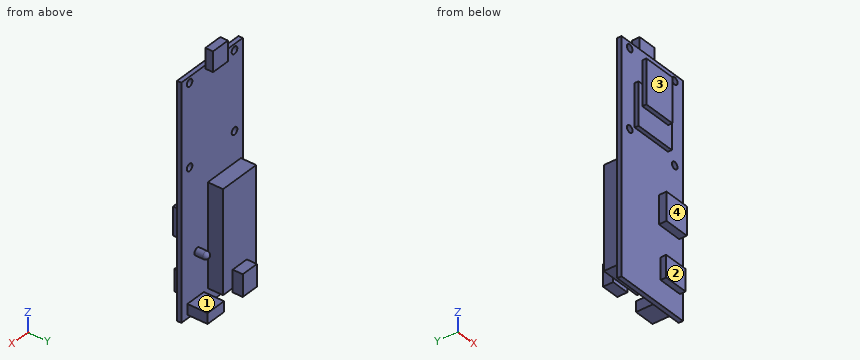
Autodesk Inventor part; units mm, degrees
ref_plane "YZ Plane" through (0, 0, 0) normal (1, 0, 0) x (0, 1, 0)
ref_plane "XZ Plane" through (0, 0, 0) normal (0, 1, 0) x (-1, 0, 0)
ref_plane "XY Plane" through (0, 0, 0) normal (0, 0, 1) x (1, 0, 0)
sketch "Sketch1" plane through (0, 0, 0) normal (0, 1, 0) x (-1, 0, 0)
  line L0 (16.375, 48.6) -> (-16.375, 48.6)
  line L1 (-16.375, 48.6) -> (-16.375, -48.6)
  line L2 (-16.375, -48.6) -> (16.375, -48.6)
  line L3 (16.375, -48.6) -> (16.375, 48.6)
  line L4 (16.375, 48.6) -> (-16.375, -48.6) construction
  line L5 (-16.375, 48.6) -> (16.375, -48.6) construction
  point P0 (0, 0)
  dimension "d0" = 32.75
  dimension "d1" = 97.2
extrude "Extrusion1" add sketch "Sketch1" along normal blind 1.8
sketch "Sketch4" plane through (0, 0, 0) normal (0, -1, 0) x (1, 0, 0)
  line L0 (8.375, 33.45) -> (-9.375, 33.45)
  line L1 (-9.375, 33.45) -> (-9.375, 15.45)
  line L2 (-9.375, 15.45) -> (8.375, 15.45)
  line L3 (8.375, 15.45) -> (8.375, 33.45)
  line L4 (16.375, 48.6) -> (16.375, -48.6)
  line L5 (-16.375, 48.6) -> (16.375, 48.6)
  point P0 (0, 0)
  dimension "d12" = 18
  dimension "d13" = 17.75
  dimension "d14" = 8
  dimension "d15" = 15.15
extrude "Extrusion4" add sketch "Sketch4" along normal blind 3.43 from surface at -1.8
sketch "Sketch5" plane through (-9.375, -1.63, 33.45) normal (0, -1, 0) x (1, 0, 0)
  line L0 (2, -9) -> (15.8, -9)
  line L1 (15.8, -9) -> (15.8, 9.6)
  line L2 (15.8, 9.6) -> (2, 9.6)
  line L3 (2, 9.6) -> (2, -9)
  line L4 (0, 0) -> (0, -18)
  line L5 (0, -18) -> (17.75, -18)
  point P0 (9.375, -33.45)
  dimension "d18" = 18.6
  dimension "d19" = 13.8
  dimension "d20" = 2
  dimension "d21" = 9
extrude "Extrusion5" add sketch "Sketch5" along normal blind 1.75 from surface at 0
sketch "Sketch6" plane through (0, 0, 0) normal (0, -1, 0) x (1, 0, 0)
  line L0 (14.375, -4.75) -> (3.525, -4.75)
  line L1 (3.525, -4.75) -> (3.525, -16.6)
  line L2 (3.525, -16.6) -> (14.375, -16.6)
  line L3 (14.375, -16.6) -> (14.375, -4.75)
  line L4 (16.375, 48.6) -> (16.375, -48.6)
  line L5 (16.375, -48.6) -> (-16.375, -48.6)
  point P0 (0, 0)
  dimension "d24" = 11.85
  dimension "d25" = 10.85
  dimension "d26" = 2
  dimension "d27" = 32
extrude "Extrusion6" add sketch "Sketch6" along normal blind 5.04 from surface at -1.8
sketch "Sketch7" plane through (0, 0, 0) normal (0, -1, 0) x (1, 0, 0)
  line L0 (14.775, -29.45) -> (4.445, -29.45)
  line L1 (4.445, -29.45) -> (4.445, -38.6)
  line L2 (4.445, -38.6) -> (14.775, -38.6)
  line L3 (14.775, -38.6) -> (14.775, -29.45)
  line L4 (16.375, 48.6) -> (16.375, -48.6)
  line L5 (16.375, -48.6) -> (-16.375, -48.6)
  point P0 (0, 0)
  dimension "d30" = 9.15
  dimension "d31" = 10.33
  dimension "d32" = 1.6
  dimension "d33" = 10
extrude "Extrusion7" add sketch "Sketch7" along normal blind 4.18 from surface at -1.8
sketch "Sketch8" plane through (0, 1.8, 0) normal (0, 1, 0) x (1, 0, 0)
  line L0 (-4.375, -47.18) -> (3.555, -47.18)
  line L1 (3.555, -47.18) -> (3.555, -55.6)
  line L2 (3.555, -55.6) -> (-4.375, -55.6)
  line L3 (-4.375, -55.6) -> (-4.375, -47.18)
  line L4 (-16.375, 48.6) -> (-16.375, -48.6)
  line L5 (-16.375, -48.6) -> (16.375, -48.6)
  point P0 (0, 0)
  dimension "d36" = 8.42
  dimension "d37" = 7.93
  dimension "d38" = 12
  dimension "d39" = 7
extrude "Extrusion8" add sketch "Sketch8" along normal blind 3.23
sketch "Sketch9" plane through (0, 1.8, 0) normal (0, 1, 0) x (1, 0, 0)
  circle A0 centre (-11.975, -46.1) radius 1.5
  circle A1 centre (11.975, -46.1) radius 1.5
  circle A2 centre (11.975, -11.9) radius 1.5
  circle A3 centre (-11.975, -13.4) radius 1.5
  line L0 (-13.475, -13.4) -> (-16.375, -13.4)
  line L1 (-16.375, 48.6) -> (-16.375, -48.6)
  line L2 (-13.475, -13.4) -> (-11.975, -13.4) construction
  line L3 (-11.975, -46.1) -> (-13.475, -46.1) construction
  line L4 (-13.475, -46.1) -> (-16.375, -46.1)
  line L5 (-11.975, -46.1) -> (-11.975, -47.6) construction
  line L6 (-16.375, -48.6) -> (16.375, -48.6)
  line L7 (-11.975, -47.6) -> (-11.975, -48.6)
  line L8 (11.975, -46.1) -> (13.475, -46.1) construction
  line L9 (13.475, -46.1) -> (16.375, -46.1)
  line L10 (11.975, -46.1) -> (11.975, -47.6) construction
  line L11 (11.975, -47.6) -> (11.975, -48.6)
  line L12 (16.375, -48.6) -> (16.375, 48.6)
  line L13 (11.975, -46.1) -> (11.975, -44.6) construction
  line L14 (11.975, -44.6) -> (11.975, -13.4)
  line L15 (11.975, -13.4) -> (11.975, -11.9) construction
  line L16 (-11.975, -46.1) -> (-11.975, -14.9)
  line L17 (-11.975, -13.4) -> (-11.975, -14.9) construction
  point P0 (0, 0)
  dimension "d42" = 3
  dimension "d43" = 2.9
  dimension "d44" = 2.9
  dimension "d45" = 1
  dimension "d46" = 1
  dimension "d47" = 2.9
  dimension "d48" = 31.2
  dimension "d49" = 31.2
extrude "Extrusion9" cut sketch "Sketch9" against normal through all contours A0 | A2 | A3 | A1
sketch "Sketch10" plane through (0, 1.8, 0) normal (0, 1, 0) x (1, 0, 0)
  line L0 (2.275, -0.55) -> (-15.375, -0.55)
  line L1 (-15.375, -0.55) -> (-15.375, 42.35)
  line L2 (-15.375, 42.35) -> (2.275, 42.35)
  line L3 (2.275, 42.35) -> (2.275, -0.55)
  line L4 (-16.375, 48.6) -> (-16.375, -48.6)
  line L5 (16.375, 48.6) -> (-16.375, 48.6)
  point P0 (0, 0)
  dimension "d52" = 42.9
  dimension "d53" = 17.65
  dimension "d54" = 1
  dimension "d55" = 6.25
extrude "Extrusion10" add sketch "Sketch10" along normal blind 6.45
sketch "Sketch11" plane through (0, 8.25, 0) normal (0, 1, 0) x (1, 0, 0)
  line L0 (-10.375, 34.85) -> (-2.855, 34.85)
  line L1 (-2.855, 34.85) -> (-2.855, 44.05)
  line L2 (-2.855, 44.05) -> (-10.375, 44.05)
  line L3 (-10.375, 44.05) -> (-10.375, 34.85)
  line L4 (2.275, 42.35) -> (-15.375, 42.35)
  line L5 (-15.375, 42.35) -> (-15.375, -0.55)
  point P0 (0, 0)
  dimension "d58" = 9.2
  dimension "d59" = 7.52
  dimension "d60" = 7.5
  dimension "d61" = 5
extrude "Extrusion11" add sketch "Sketch11" along normal blind 4.25
sketch "Sketch12" plane through (0, 1.8, 0) normal (0, 1, 0) x (1, 0, 0)
  circle A0 centre (7.875, 24.35) radius 1.5
  line L0 (7.875, 24.35) -> (9.375, 24.35) construction
  line L1 (9.375, 24.35) -> (16.375, 24.35)
  line L2 (16.375, -48.6) -> (16.375, 48.6)
  line L3 (7.875, 24.35) -> (7.875, 25.85) construction
  line L4 (7.875, 25.85) -> (7.875, 48.6)
  line L5 (16.375, 48.6) -> (-16.375, 48.6)
  point P0 (0, 0)
  dimension "d64" = 3
  dimension "d65" = 7
  dimension "d66" = 22.75
extrude "Extrusion12" add sketch "Sketch12" along normal blind 5 contours A0
fillet "Fillet1" radius 1.5 1 edges at (6.375, 6.8, -24.35)
sketch "Sketch13" plane through (0, 1.8, 0) normal (0, 1, 0) x (1, 0, 0)
  line L0 (13.125, 47.1) -> (4.375, 47.1)
  line L1 (4.375, 47.1) -> (4.375, 42.7)
  line L2 (4.375, 42.7) -> (13.125, 42.7)
  line L3 (13.125, 42.7) -> (13.125, 47.1)
  line L4 (16.375, 48.6) -> (-16.375, 48.6)
  line L5 (16.375, -48.6) -> (16.375, 48.6)
  point P0 (0, 0)
  dimension "d70" = 8.75
  dimension "d71" = 4.4
  dimension "d72" = 1.5
  dimension "d73" = 3.25
extrude "Extrusion13" add sketch "Sketch13" along normal blind 10.3 from surface at -1.8
properties part number "PCB Board"
Build history of the part. All positions in model axes, mm. Face numbers are marked on the shaded views. A direction names the side the tool comes from. Give positions to 0.01 mm unless a question says otherwise; leave off trailing zeros. Write each loop counter-clockwise with the first axis right and the second up, starting at its lowest first coordinate (ties: lowest second). Pieces come first, ordered by that corner, then holes. Notation, with made-up numbers: (10.5, 68.5) - (15.5, 68.5) arc R19 cw to (15.5, 101.5) - close; hole circle Ø3 at (72.5, -20). An arc over 180 degrees is marked (long way). Use one line per item in the form item = value. Start each with the question number.
1. Band-saw the part on A-A on z = 46.1. Write the cut outline in (x, y) (3 decimals), plus the area to 4 significant figures.
2. Band-saw the part on D-D on x = -11.5. Write the cut outline in (y, z).
3. Probe line 1 (X direction, y = 0.4, z = 46.1) (3 decimals); line 2 (Y direction, x = 5.5, z = 36.5); line 3 (Y direction, x = -11, z = -30.5). List the from-to ranges inside material, lowest first. Write a range as [from, to].
4. Two-plate mould, pull along Z, no slides. Class the marked faces 1 and 2: released by +Z, released by -Z, zero draft, split by the parting line, or undercut.
5. Drop flat-ended pins along their axis: pin 1 Ø4 at (x, z) = (3.5, 0.5) entering from +Y; pin 2 Ø1 at (y, z) = (-1.5, -13.5) entering from -X (3 decimals); pin 3 Ø1.9 at (x, y) = (11, -1.5) entering from -Z; pin 4 Ø2.5 at (x, z) = (11.975, 46.1) entering from +Y. Give the stop position or say it passes through.
6. Band-saw the part on B-B on y = 3.75. Write the cut outline in (x, z) (3 decimals), plus the area to 3 significant figures.
7. Band-saw the part on C-C on z = -24.35. Write the cut outline in (x, y) (3 decimals).
8. 3-axis set-ups, long thin cutter, end or side, ignore diameter. For the marked faces 3 and 4: which of +Z, -Z, +X, -X, +Y, -Y reach the whole face in a straight line?
Conclusion:
q1.outline = (-16.375, 0) - (-13.475, 0) - (-13.475, 1.8) - (-16.375, 1.8) - close; (-10.475, 0) - (10.475, 0) - (10.475, 1.8) - (-10.475, 1.8) - close; (13.475, 0) - (16.375, 0) - (16.375, 1.8) - (13.475, 1.8) - close
q1.area = 48.15 mm²
q2.outline = (0, -48.6) - (1.8, -48.6) - (1.8, -42.35) - (8.25, -42.35) - (8.25, 0.55) - (1.8, 0.55) - (1.8, 11.98) - (0, 11.98) - close; (0, 14.82) - (1.8, 14.82) - (1.8, 44.68) - (0, 44.68) - close; (0, 47.52) - (1.8, 47.52) - (1.8, 48.6) - (0, 48.6) - close
q3.line_1 = [-16.375, -13.475], [-10.475, 10.475], [13.475, 16.375]
q3.line_2 = [-3.38, -1.63], [0, 1.8]
q3.line_3 = [0, 8.25]
q4.face_1 = undercut
q4.face_2 = zero draft
q5.pin_1 = 8.25
q5.pin_2 = 3.525
q5.pin_3 = -38.6
q5.pin_4 = through
q6.outline = (-15.375, -42.35) - (2.275, -42.35) - (2.275, 0.55) - (-15.375, 0.55) - close; (-4.375, 47.18) - (3.555, 47.18) - (3.555, 55.6) - (-4.375, 55.6) - close; (4.375, -47.1) - (13.125, -47.1) - (13.125, -42.7) - (4.375, -42.7) - close; circle Ø3 at (7.875, -24.35)
q6.area = 870 mm²
q7.outline = (-16.375, 0) - (16.375, 0) - (16.375, 1.8) - (9.375, 1.8) - (9.375, 5.3) arc R1.5 ccw to (6.375, 5.3) - (6.375, 1.8) - (2.275, 1.8) - (2.275, 8.25) - (-15.375, 8.25) - (-15.375, 1.8) - (-16.375, 1.8) - close
q8.face_3 = +Z, -Z, +X, -X, -Y
q8.face_4 = -Z, +X, -X, -Y
